from build123d import *

# Parameters (mm, degrees)
SKETCH_1_R          = 8
SKETCH_1_R_2        = 1.5
EXTRUDE_1_DEPTH     = 5
SKETCH_2_R          = 1.5
CUT_EXTRUDE_1_DEPTH = 11.5


with BuildPart() as part:
    # 草图1 → 凸台-拉伸1 (new body)
    with BuildSketch(Plane.XY):
        with BuildLine():
            Line((2.5, 15), (8.5, 15))
            ThreePointArc((8.5, 15), (10.267766953, 15.732233047), (11, 17.5))
            Line((11, 17.5), (11, 18))
            ThreePointArc((11, 18), (12.171572875, 20.828427125), (15, 22))
            Line((15, 22), (42, 22))
            ThreePointArc((42, 22), (44.828427125, 20.828427125), (46, 18))
            Line((46, 18), (46, 17.5))
            ThreePointArc((46, 17.5), (46.732233047, 15.732233047), (48.5, 15))
            Line((48.5, 15), (54.5, 15))
            ThreePointArc((54.5, 15), (56.267766953, 14.267766953), (57, 12.5))
            Line((57, 12.5), (57, 9.5))
            ThreePointArc((57, 9.5), (56.267766953, 7.732233047), (54.5, 7))
            Line((54.5, 7), (48.5, 7))
            ThreePointArc((48.5, 7), (46.732233047, 6.267766953), (46, 4.5))
            Line((46, 4.5), (46, 4))
            ThreePointArc((46, 4), (44.828427125, 1.171572875), (42, 0))
            Line((42, 0), (15, 0))
            ThreePointArc((15, 0), (12.171572875, 1.171572875), (11, 4))
            Line((11, 4), (11, 4.5))
            ThreePointArc((11, 4.5), (10.267766953, 6.267766953), (8.5, 7))
            Line((8.5, 7), (2.5, 7))
            ThreePointArc((2.5, 7), (0.732233047, 7.732233047), (0, 9.5))
            Line((0, 9.5), (0, 12.5))
            ThreePointArc((0, 12.5), (0.732233047, 14.267766953), (2.5, 15))
        make_face()
        with Locations((28.5, 11)):
            Circle(SKETCH_1_R, mode=Mode.SUBTRACT)
        with Locations((15, 18)):
            Circle(SKETCH_1_R_2, mode=Mode.SUBTRACT)
        with Locations(Location((15, 4, 0), (0, 0, 180))):
            Circle(SKETCH_1_R_2, mode=Mode.SUBTRACT)
        with Locations(Location((42, 18, 0), (0, 0, 180))):
            Circle(SKETCH_1_R_2, mode=Mode.SUBTRACT)
        with Locations((42, 4)):
            Circle(SKETCH_1_R_2, mode=Mode.SUBTRACT)
        with Locations((3, 11)):
            Circle(SKETCH_1_R_2, mode=Mode.SUBTRACT)
        with Locations(Location((54, 11, 0), (0, 0, 180))):
            Circle(SKETCH_1_R_2, mode=Mode.SUBTRACT)
    extrude(amount=EXTRUDE_1_DEPTH)

    # 草图2 → 切除-拉伸1 (cut)
    with BuildSketch(Plane(origin=(0, 15, 0), x_dir=(1, 0, 0), z_dir=(0, 1, 0))):
        with Locations((7, -5)):
            Circle(SKETCH_2_R)
        with Locations((50, -5)):
            Circle(SKETCH_2_R)
    extrude(amount=-CUT_EXTRUDE_1_DEPTH, mode=Mode.SUBTRACT)


solid = part.part
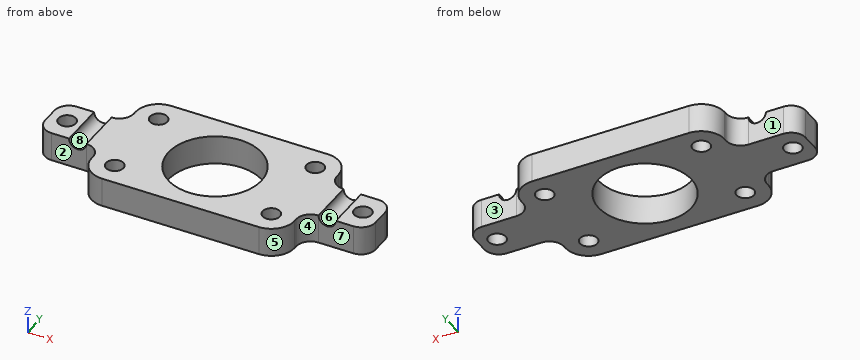
Input: part model. Units: mm. Frame: model coordinates. Face numbers are marked on the shaded views. A direction names the side the tool comes from. Coordinates: 2 decimals unless noted, no trailing zeros. Loops run counter-clockwise (first coordinate to the right, second up) from the corner with the lowest first, then second, coordinate; pieces in that order, holes last. Notation, with made-up numbers: (28, -7) -> (46, -7) arc R15 cw to (46, 10) -> close; hole circle Ø11 at (-9.5, 26.25). An arc over 180 degrees is marked (long way). Write each question's results on one line, items separated by ' | '. Start each with the question number.
Q1. Ray query, line 1 (Y direction, x = 42, z = 3.4); line 2 (X direction, y = 11.25, z = 2.85); line 3 (Y direction, x = 3, z = 3.9). Return the intervals inside material, ascending. Write a range as from..to.
Q2. Pin query (flat end, axial travel): pin 1 (2 mm diameter, centred on y = 18, z = 3, fed in from +X); pin 2 (1 mm diameter, centred on y = 3, z = 3.5, fed in from -X); pin 3 (1.5 mm diameter, centred on x = 51, z = 1.5, fed in from +Y). Return the tip coordinate at first contact, or that it passes through.
Q3. Pull-direction query (X, two-part tool) for the marked faces 5, 6, 7 and 8; classes: released by +X, released by -X, zero draft, split by the parting line, or undercut.
Q4. Reachability of the marked faces 1, 2, 3 and 4 from +Z, -Z, +X, -X, +Y, -Y: full face, straight path, thin tool, end or side. Return the list, or none.
Q5. Section D-D, the plane x = 3. Return the cut outline in (y, z).
Q6. Section C-C, the plane y = 10.5. Return the cut outline in (x, z).
Q7. Section A-A, the plane x = 28.5. Return the cut outline in (y, z).
Q8. Section B-B, the plane z = 1. State how many separate pieces and enclosed holes the cut face has, plus the area to 3 significant figures.
Found:
1) line 1: 0..2.5, 5.5..16.5, 19.5..22 | line 2: 0..1.52, 4.48..20.5, 36.5..52.52, 55.48..57 | line 3: 7..9.5, 12.5..15
2) pin 1: x = 46.05 | pin 2: x = 11.03 | pin 3: y = 15
3) face 5: released by +X | face 6: undercut | face 7: zero draft | face 8: undercut
4) face 1: +Z, -Z, -X, +Y | face 2: +Z, -Z, -X, -Y | face 3: +Z, -Z, +X, +Y | face 4: +Z, -Z, +X, -Y
5) outline: (7, 0) -> (9.5, 0) -> (9.5, 5) -> (7, 5) -> close; (12.5, 0) -> (15, 0) -> (15, 5) -> (12.5, 5) -> close
6) outline: (0, 0) -> (1.59, 0) -> (1.59, 5) -> (0, 5) -> close; (4.41, 0) -> (20.52, 0) -> (20.52, 5) -> (8.5, 5) arc R1.5 cw to (5.5, 5) -> (4.41, 5) -> close; (36.48, 0) -> (52.59, 0) -> (52.59, 5) -> (51.5, 5) arc R1.5 cw to (48.5, 5) -> (36.48, 5) -> close; (55.41, 0) -> (57, 0) -> (57, 5) -> (55.41, 5) -> close
7) outline: (0, 0) -> (3, 0) -> (3, 5) -> (0, 5) -> close; (19, 0) -> (22, 0) -> (22, 5) -> (19, 5) -> close
8) separate pieces: 1 | enclosed holes: 7 | area: 689 mm2
